Verification items for the finished model (mm, model axes). A direction names the side the tool comes from. Coordinates: 2 decimals unless noted, no trailing zeros. Write each loop counter-clockwise with the first axis right and the second up, starting at its lowest first coordinate (ties: lowest second). Pieces come first, ordered by that corner, then holes.
```python
from build123d import *

# Parameters (mm, degrees)
REVOLVE1_ANGLE = 352


with BuildPart() as part:
    # Sketch1 → Revolve1 (revolve)
    with BuildSketch(Plane(origin=(0, 0, 0), x_dir=(1, 0, 0), z_dir=(0, 1, 0))):
        with BuildLine():
            Line((11, 10.35), (11, 1))
            ThreePointArc((11, 1), (11.292893219, 0.292893219), (12, 0))
            Line((12, 0), (12.782227205, 0))
            ThreePointArc((12.782227205, 0), (13.770601827, 0.409398173), (14.18, 1.397772795))
            Line((14.18, 1.397772795), (12.75, 1.397772795))
            Line((12.75, 1.397772795), (12.75, 10.35))
            Line((12.75, 10.35), (11, 10.35))
        make_face()
    revolve(axis=Axis((0, 0, 0), (0, 0, -1)), revolution_arc=REVOLVE1_ANGLE)


solid = part.part
```
1. Tool access check on faces 4 (the flat face through (-12, -5, -1.398)), 5 (the flat face through (12, 0, -5)). Record the directions out of +Z, -Z, +X, -X, +Y, -Y that give a thin tool (end or side, any length) a straight path to the whole face; none if there is none.
2. Gauge pin test, flat ends, axial feed: P1, Ø12, axis at x = 7, y = 7.5, coming from the +Z side; P2, Ø1.5, axis at x = -6, y = 6.5, coming from the +Z side; P3, Ø1, axis at y = 10.5, z = -3.5, coming from the +X side; P4, Ø4, axis at x = -1, z = -6, coming from the -Y side. Record the tip position at first contact, or that the pin passes through.
3. Material ranges on L1, parallel to Y at x = 0, z = -5.5; L2, parallel to Y at x = 8.75, z = -3.5; L3, parallel to X at y = 8.5, z = -5.5, recorded low to high.
4. Draft check along Y on faces 1 (the flat face through (-6, -10, -10.35)), 2 (the cylindrical face through (-10.93, -1.24, -5.61)), 3 (the cylindrical face through (-12.67, -1.44, -5.94)). Enter one of: pulls with the +Y half, pulls with the -Y half, needs draft (parallel to the pull), parting line crosses it, or undercut.
5. Sectioned sample at A-A, the plane x = 0. Record the boundary of the cut face in (y, z), and give its area (3 significant figures).
6. Sectioned sample at B-B, the plane z = -9.5. Record the boundary of the cut face in (x, y).
Outcome:
1. face 4: -Z
1. face 5: +Z, -Z, +X
2. P1: stops at z = 0
2. P2: passes through
2. P3: stops at x = 7.91
2. P4: stops at y = -12.75
3. L1: y = -12.75 to -11, 11 to 12.75
3. L2: y = -9.27 to -6.67, 6.67 to 9.27
3. L3: x = -9.5 to -6.98, 6.98 to 9.5
4. face 1: needs draft
4. face 2: undercut
4. face 3: parting line crosses it
5. outline: (-14.18, -1.4) - (-12.75, -1.4) - (-12.75, -10.35) - (-11, -10.35) - (-11, -1) arc R1 ccw to (-12, 0) - (-12.78, 0) arc R1.4 ccw to start; (11, -10.35) - (12.75, -10.35) - (12.75, -1.4) - (14.18, -1.4) arc R1.4 ccw to (12.78, 0) - (12, 0) arc R1 ccw to (11, -1) - close
5. area: 39.0 mm2
6. outline: (10.89, 1.53) - (12.63, 1.77) arc R12.75 ccw (long way) to (12.75, 0) - (11, 0) arc R11 cw (long way) to start
